Check sheet for the modelled part. Datum: model origin and axes. Units: mm. A direction names the side the tool comes from. Coordinates: 2 decimals unless noted, no trailing zeros. Order: outer loops, then holes, each group sorted by start corner. A loop starts at its lowest first (then second) coordinate and runs counter-clockwise, first axis right, second up.
1. Draft check along Y on faces 1 (the flat face through (-1, 7, -3.25)), 2 (the cylindrical face through (-2.38, -10.74, 0.05)), 3 (the flat face through (-3, 3, -3.5)). Enter one of: released by +Y, released by -Y, zero draft, split by the parting line, or undercut.
2. Thickness scan on line 1 (Y direction, x = 0, z = 1); line 2 (Z direction, x = 4.25, y = 6.5); line 3 (Y direction, x = -1.75, z = 2). Record the ranges inside material, lowest first.
3. Cross-section at A-A (y = 0). Enter the section's corners in (x, z).
4. Set-up check for faces 4 (the flat face through (3, 3, 3.5)), 5 (the flat face through (1, 7, 3.25)): record each of +Z, -Z, +X, -X, +Y, -Y from which the full face is reachable in a straight line by a thin tool's end or side.
5. Cross-section at C-C (z = -2.5). Enter the section's corners in (x, y), then the cut area to 3 significant figures.
```python
from build123d import *

# Parameters (mm, degrees)
CHAMFER_SIZE = 0.25


with BuildPart() as part:
    # Sketch001 → Revolution (revolve)
    with BuildSketch(Plane.XZ):
        Polygon((4, -3.5), (6.5, -3.5), (6.75, -3.25), (9, -3.25), (9.25, -3.5), (11, -3.5), (11, 3.5), (9.25, 3.5), (9, 3.25), (6.75, 3.25), (6.5, 3.5), (4, 3.5), align=None)
    revolve(axis=Axis((0, 0, 0), (0, 0, 1)))

    # Chamfer
    chamfer_edges = [part.edges().sort_by_distance(p)[0] for p in [
        (-11, 0, 3.5),
        (-11, 0, -3.5),
    ]]
    chamfer(chamfer_edges, length=CHAMFER_SIZE)


solid = part.part
```
Data:
1. face 1: undercut
1. face 2: split by the parting line
1. face 3: zero draft
2. line 1: y = -11 to -4, 4 to 11
2. line 2: z = -3.25 to 3.25
2. line 3: y = -10.86 to -3.6, 3.6 to 10.86
3. outline: (-11, -3.25) - (-10.75, -3.5) - (-9.25, -3.5) - (-9, -3.25) - (-6.75, -3.25) - (-6.5, -3.5) - (-4, -3.5) - (-4, 3.5) - (-6.5, 3.5) - (-6.75, 3.25) - (-9, 3.25) - (-9.25, 3.5) - (-10.75, 3.5) - (-11, 3.25) - close; (4, -3.5) - (6.5, -3.5) - (6.75, -3.25) - (9, -3.25) - (9.25, -3.5) - (10.75, -3.5) - (11, -3.25) - (11, 3.25) - (10.75, 3.5) - (9.25, 3.5) - (9, 3.25) - (6.75, 3.25) - (6.5, 3.5) - (4, 3.5) - close
4. face 4: +Z, +X, -X, +Y, -Y
4. face 5: +Z
5. outline: circle Ø22 at (0, 0); hole circle Ø8 at (0, 0)
5. area: 330 mm2
